Autodesk Inventor part; units mm, degrees
ref_plane "YZ Plane" through (0, 0, 0) normal (1, 0, 0) x (0, 1, 0)
ref_plane "XZ Plane" through (0, 0, 0) normal (0, 1, 0) x (-1, 0, 0)
sketch "layer_layout_sketch" plane through (0, 0, 0) normal (0, 0, 1) x (1, 0, 0)
  line L0 (-400, 250) -> (400, 250)
  line L1 (400, 250) -> (400, -250)
  line L2 (400, -250) -> (-400, -250)
  line L3 (-400, -250) -> (-400, 250)
  line L4 (0, 250) -> (0, -250) construction
  line L5 (-400, 200) -> (400, 200)
  line L6 (400, 200) -> (400, -200)
  line L7 (400, -200) -> (-400, -200)
  line L8 (-400, -200) -> (-400, 200)
  line L9 (0, 200) -> (0, -200) construction
  line L10 (-400, 150) -> (400, 150)
  line L11 (400, 150) -> (400, -150)
  line L12 (400, -150) -> (-400, -150)
  line L13 (-400, -150) -> (-400, 150)
  line L14 (0, 150) -> (0, -150) construction
  point P0 (0, 0)
  point P1 (0, 0)
  dimension "d116" = 500
  dimension "d117" = 800
  dimension "d122" = 400
  dimension "d123" = 300
sketch "coil_layer_sketch_lower" plane through (0, 0, 0) normal (0, 0, 1) x (1, 0, 0)
  line L0 (0, -9.3) -> (376.5, -9.3)
  line L1 (395, -27.8) -> (395, -131.5)
  line L2 (376.5, -150) -> (-376.5, -150)
  line L3 (-395, -131.5) -> (-395, -50.9)
  line L4 (0, -9.3) -> (0, -13.8)
  line L5 (0, -13.8) -> (375.5, -13.8)
  line L6 (390.5, -28.8) -> (390.5, -130.5)
  line L7 (375.5, -145.5) -> (-375.5, -145.5)
  line L8 (-376.5, -32.4) -> (363.75, -32.4)
  line L9 (382.25, -50.9) -> (382.25, -118.75)
  line L10 (363.75, -137.25) -> (-363.75, -137.25)
  line L11 (-390.5, -130.5) -> (-390.5, -51.9)
  line L12 (-375.5, -36.9) -> (362.75, -36.9)
  line L13 (377.75, -51.9) -> (377.75, -117.75)
  line L14 (362.75, -132.75) -> (-362.75, -132.75)
  line L15 (-377.75, -117.75) -> (-377.75, -75)
  line L16 (-382.25, -118.75) -> (-382.25, -74)
  line L17 (-363.75, -55.5) -> (351, -55.5)
  line L18 (369.5, -74) -> (369.5, -106)
  line L19 (-362.75, -60) -> (350, -60)
  line L20 (365, -75) -> (365, -105)
  line L21 (-558.3641, 0) -> (558.3641, 0)
  line L22 (350, -120) -> (-350, -120)
  line L23 (351, -124.5) -> (-351, -124.5)
  line L24 (-369.5, -106) -> (-369.5, -71.7563)
  line L25 (-369.5, -71.7563) -> (-365, -71.7563)
  line L26 (-365, -71.7563) -> (-365, -105)
  arc A0 (395, -27.8) -> (376.5, -9.3) centre (376.5, -27.8) ccw
  arc A1 (382.25, -50.9) -> (363.75, -32.4) centre (363.75, -50.9) ccw
  arc A2 (369.5, -74) -> (351, -55.5) centre (351, -74) ccw
  arc A3 (351, -124.5) -> (369.5, -106) centre (351, -106) ccw
  arc A4 (363.75, -137.25) -> (382.25, -118.75) centre (363.75, -118.75) ccw
  arc A5 (376.5, -150) -> (395, -131.5) centre (376.5, -131.5) ccw
  arc A6 (-395, -131.5) -> (-376.5, -150) centre (-376.5, -131.5) ccw
  arc A7 (-382.25, -118.75) -> (-363.75, -137.25) centre (-363.75, -118.75) ccw
  arc A8 (-369.5, -106) -> (-351, -124.5) centre (-351, -106) ccw
  arc A9 (-376.5, -32.4) -> (-395, -50.9) centre (-376.5, -50.9) ccw
  arc A10 (-363.75, -55.5) -> (-382.25, -74) centre (-363.75, -74) ccw
  arc A11 (-375.5, -36.9) -> (-390.5, -51.9) centre (-375.5, -51.9) ccw
  arc A12 (-362.75, -60) -> (-377.75, -75) centre (-362.75, -75) ccw
  arc A13 (-390.5, -130.5) -> (-375.5, -145.5) centre (-375.5, -130.5) ccw
  arc A14 (-377.75, -117.75) -> (-362.75, -132.75) centre (-362.75, -117.75) ccw
  arc A15 (-365, -105) -> (-350, -120) centre (-350, -105) ccw
  arc A16 (350, -120) -> (365, -105) centre (350, -105) ccw
  arc A17 (362.75, -132.75) -> (377.75, -117.75) centre (362.75, -117.75) ccw
  arc A18 (375.5, -145.5) -> (390.5, -130.5) centre (375.5, -130.5) ccw
  arc A19 (377.75, -51.9) -> (362.75, -36.9) centre (362.75, -51.9) ccw
  arc A20 (390.5, -28.8) -> (375.5, -13.8) centre (375.5, -28.8) ccw
  arc A21 (365, -75) -> (350, -60) centre (350, -75) ccw
  point P0 (0, 0)
  point P1 (0, 0)
  point P2 (368.0934, -60)
  point P3 (370, -61.9066)
  point P4 (0, -150)
  dimension "d1" = 4.5
  dimension "d2" = 4.5
  dimension "d3" = 4.5
  dimension "d4" = 9.3
  dimension "d5" = 790
  dimension "d6" = 395
  dimension "d7" = 4.5
  dimension "d8" = 4.5
  dimension "d9" = 8.25
  dimension "d10" = 4.5
  dimension "d11" = 18.6
  dimension "d12" = 4.5
  dimension "d13" = 8.25
  dimension "d14" = 4.5
  dimension "d15" = 4.5
  dimension "d16" = 4.5
  dimension "d17" = 8.25
  dimension "d19" = 18.6
  dimension "d20" = 8.25
  dimension "d82" = 150
  dimension "d88" = 4.5
  dimension "d89" = 8.25
  dimension "d96" = 4.5
  dimension "d97" = 8.25
  dimension "d98" = 18.5
  dimension "d99" = 15
  dimension "d109" = 15
sketch "coil_layer_sketch_upper" plane through (0, 0, 0) normal (0, 0, 1) x (1, 0, 0)
  line L0 (0, -13.8) -> (-376.5, -13.8)
  line L1 (-395, 4.7) -> (-395, 131.5)
  line L2 (-376.5, 150) -> (376.5, 150)
  line L3 (395, 131.5) -> (395, 27.8)
  line L4 (0, -9.3) -> (-375.5, -9.3)
  line L5 (-390.5, 5.7) -> (-390.5, 130.5)
  line L6 (-375.5, 145.5) -> (375.5, 145.5)
  line L7 (390.5, 130.5) -> (390.5, 28.8)
  line L8 (375.5, 13.8) -> (-362.75, 13.8)
  line L9 (-377.75, 28.8) -> (-377.75, 117.75)
  line L10 (376.5, 9.3) -> (-363.75, 9.3)
  line L11 (-382.25, 27.8) -> (-382.25, 118.75)
  line L12 (-362.75, 132.75) -> (362.75, 132.75)
  line L13 (-363.75, 137.25) -> (363.75, 137.25)
  line L14 (377.75, 117.75) -> (377.75, 51.9)
  line L15 (362.75, 36.9) -> (-350, 36.9)
  line L16 (382.25, 118.75) -> (382.25, 50.9)
  line L17 (363.75, 32.4) -> (-351, 32.4)
  line L18 (-365, 51.9) -> (-365, 105)
  line L19 (-350, 120) -> (350, 120)
  line L20 (365, 105) -> (365, 75)
  line L21 (350, 60) -> (-356.75, 60)
  line L22 (-369.5, 50.9) -> (-369.5, 106)
  line L23 (-351, 124.5) -> (351, 124.5)
  line L24 (369.5, 106) -> (369.5, 74)
  line L25 (351, 55.5) -> (-356.75, 55.5)
  line L26 (-356.75, 60) -> (-356.75, 55.5)
  line L27 (-700, 0) -> (700, 0)
  line L28 (-980, 0) -> (980, 0)
  line L29 (0, -13.8) -> (0, -9.3)
  line L30 (0, -51.9241) -> (0, 188.1241)
  arc A0 (365, 105) -> (350, 120) centre (350, 105) ccw
  arc A1 (350, 60) -> (365, 75) centre (350, 75) ccw
  arc A2 (377.75, 117.75) -> (362.75, 132.75) centre (362.75, 117.75) ccw
  arc A3 (362.75, 36.9) -> (377.75, 51.9) centre (362.75, 51.9) ccw
  arc A4 (390.5, 130.5) -> (375.5, 145.5) centre (375.5, 130.5) ccw
  arc A5 (375.5, 13.8) -> (390.5, 28.8) centre (375.5, 28.8) ccw
  arc A6 (-350, 120) -> (-365, 105) centre (-350, 105) ccw
  arc A7 (-365, 51.9) -> (-350, 36.9) centre (-350, 51.9) ccw
  arc A8 (-377.75, 28.8) -> (-362.75, 13.8) centre (-362.75, 28.8) ccw
  arc A9 (-390.5, 5.7) -> (-375.5, -9.3) centre (-375.5, 5.7) ccw
  arc A10 (-362.75, 132.75) -> (-377.75, 117.75) centre (-362.75, 117.75) ccw
  arc A11 (-375.5, 145.5) -> (-390.5, 130.5) centre (-375.5, 130.5) ccw
  arc A12 (-376.5, 150) -> (-395, 131.5) centre (-376.5, 131.5) ccw
  arc A13 (-363.75, 137.25) -> (-382.25, 118.75) centre (-363.75, 118.75) ccw
  arc A14 (-351, 124.5) -> (-369.5, 106) centre (-351, 106) ccw
  arc A15 (-369.5, 50.9) -> (-351, 32.4) centre (-351, 50.9) ccw
  arc A16 (-382.25, 27.8) -> (-363.75, 9.3) centre (-363.75, 27.8) ccw
  arc A17 (-395, 4.7) -> (-376.5, -13.8) centre (-376.5, 4.7) ccw
  arc A18 (351, 55.5) -> (369.5, 74) centre (351, 74) ccw
  arc A19 (363.75, 32.4) -> (382.25, 50.9) centre (363.75, 50.9) ccw
  arc A20 (376.5, 9.3) -> (395, 27.8) centre (376.5, 27.8) ccw
  arc A21 (395, 131.5) -> (376.5, 150) centre (376.5, 131.5) ccw
  arc A22 (382.25, 118.75) -> (363.75, 137.25) centre (363.75, 118.75) ccw
  arc A23 (369.5, 106) -> (351, 124.5) centre (351, 106) ccw
  point P0 (0, 0)
  point P1 (395, 9.3)
  point P2 (-382.25, 9.3)
  point P3 (0, 150)
  point P4 (-700, 0)
  point P5 (700, 0)
  point P6 (0, 150)
  dimension "d58" = 4.5
  dimension "d59" = 4.5
  dimension "d60" = 4.5
  dimension "d61" = 8.25
  dimension "d62" = 8.25
  dimension "d64" = 4.5
  dimension "d65" = 4.5
  dimension "d66" = 4.5
  dimension "d67" = 8.25
  dimension "d69" = 18.6
  dimension "d70" = 4.5
  dimension "d71" = 4.5
  dimension "d72" = 18.6
  dimension "d73" = 8.25
  dimension "d74" = 8.25
  dimension "d75" = 4.5
  dimension "d77" = 18.6
  dimension "d78" = 4.5
  dimension "d79" = 4.5
  dimension "d80" = 4.5
  dimension "d83" = 150
  dimension "d87" = 8.25
  dimension "d91" = 4.5
  dimension "d92" = 9.3
  dimension "d93" = 790
  dimension "d100" = 15
  dimension "d101" = 18.5
  dimension "d102" = 8.25
extrude "layer_sheet Extrude" add sketch "layer_layout_sketch" along normal blind 4.5
extrude "wire_holes_upper Cut" cut sketch "coil_layer_sketch_upper" along normal blind 4.5 contours L0 A17 L27 A9 L4 L29 | A17 L1 A12 L2 L30 L6 A11 L5 A9 L27 | L30 L8 A5 L7 A4 L6 L2 A21 L3 A20 L10 | L10 A16 L11 A13 L13 L30 L12 A10 L9 A8 L8 | L30 L15 A3 L14 A2 L12 L13 A22 L16 A19 L17 | L17 A15 L22 A14 L23 L30 L19 A6 L18 A7 L15 | L30 L21 A1 L20 A0 L19 L23 A23 L24 A18 L25 | L25 L26 L21 L30
extrude "wire_holes_lower Cut" cut sketch "coil_layer_sketch_lower" along normal blind 4.5
sketch "Sketch6" plane through (0, 0, 4.5) normal (0, 0, 1) x (1, 0, 0)
  circle A0 centre (-353, 57.75) radius 3
  line L0 (400, 250) -> (-400, 250)
  line L1 (-400, 250) -> (-400, -250)
  line L2 (-400, -250) -> (400, -250)
  circle A1 centre (-353, -122) radius 3
  point P0 (0, 0)
  dimension "d124" = 6
  dimension "d125" = 192.25
  dimension "d126" = 47
  dimension "d130" = 6
  dimension "d131" = 128
  dimension "d132" = 47
equation "\"d1\" = wire_diameter"
equation "\"d2\" = wire_diameter"
equation "\"d3\" = wire_diameter"
equation "\"d4\" = 0.5 * distance_between_wires"
equation "\"d7\" = wire_diameter"
equation "\"d8\" = wire_diameter"
equation "\"d9\" = distance_between_wires_edge"
equation "\"d10\" = wire_diameter"
equation "\"d11\" = distance_between_wires"
equation "\"d12\" = wire_diameter"
equation "\"d13\" = distance_between_wires_edge"
equation "\"d14\" = wire_diameter"
equation "\"d15\" = wire_diameter"
equation "\"d16\" = wire_diameter"
equation "\"d17\" = distance_between_wires_edge"
equation "\"d19\" = distance_between_wires"
equation "\"d20\" = distance_between_wires_edge"
equation "\"d82\" = 0.5 * track_width"
equation "\"d58\" = wire_diameter"
equation "\"d59\" = wire_diameter"
equation "\"d60\" = wire_diameter"
equation "\"d61\" = distance_between_wires_edge"
equation "\"d62\" = distance_between_wires_edge"
equation "\"d64\" = wire_diameter"
equation "\"d65\" = wire_diameter"
equation "\"d66\" = wire_diameter"
equation "\"d67\" = distance_between_wires_edge"
equation "\"d69\" = distance_between_wires"
equation "\"d70\" = wire_diameter"
equation "\"d71\" = wire_diameter"
equation "\"d72\" = distance_between_wires"
equation "\"d73\" = distance_between_wires_edge"
equation "\"d74\" = distance_between_wires_edge"
equation "\"d75\" = wire_diameter"
equation "\"d77\" = distance_between_wires"
equation "\"d78\" = wire_diameter"
equation "\"d79\" = wire_diameter"
equation "\"d80\" = wire_diameter"
equation "\"d83\" = 0.5 * track_width"
equation "\"wire_diameter\" = 4.5"
equation "\"distance_between_wires\" = -1.2 * wire_diameter + 0.2 * parameter_6"
equation "\"distance_between_wires_edge\" = 8.25"
equation "\"bend_radius_inner\" = 15"
equation "\"bend_radius_outer\" = 18.5"
properties part number "primary_coil_0R2"
Verification items for the finished model (mm, model axes). Give positions to 0.01 mm unless a question says otherwise; leave off trailing zeros.
(1) Mould release check, pull along Y, two halves, no side actions. Record for faces 1 (the face through (373.24, 128.47, 2.22)), 2 (the face through (-6, 4, 0)): +Y half, -Y half, draft (parallel to the pull), parting line (faces both ways), or undercut.
(2) Material ranges on line 1 (X direction, y = 4, z = 2.6); line 2 (X direction, y = -133, z = 3.65), recorded low to high.
(3) Cross-section at A-A (x = -108). State how many separate pieces and enclosed holes the cut face has, plus the area to 3 significant figures.
Worked out:
1. face 1: undercut
1. face 2: draft
2. line 1: x = -400 to -394.99, -390.4 to 400
2. line 2: x = -400 to -394.94, -390.29 to -375.55, 375.55 to 390.29, 394.94 to 400
3. separate pieces: 13
3. enclosed holes: 0
3. area: 2,010 mm2
